CAD build for the part. Positions are in the model's coordinates, mm. A direction names the side the tool comes from. Coordinates: 2 decimals unless noted, no trailing zeros. Loops run counter-clockwise (first coordinate to the right, second up) from the corner with the lowest first, then second, coordinate; pieces in that order, holes last. Notation, with made-up numbers: (0, 20) -> (37, 20) arc R8 ccw to (37, 31) -> close; hole circle Ø5 at (20.5, -36.5). An arc over 180 degrees is marked (long way). Write each question's results on one line, items separated by ' | '.
from build123d import *

# Parameters (mm, degrees)
CROQUIS1_R              = 1.5
SALIENTE_EXTRUIR1_DEPTH = 10
CORTAR_EXTRUIR1_DEPTH   = 2
CHAFL_N2_SIZE           = 0.1
CHAFL_N3_SIZE           = 0.2
CHAFL_N3_SIZE2          = 0.346410162


with BuildPart() as part:
    # Croquis1 → Saliente-Extruir1 (new body)
    with BuildSketch(Plane(origin=(0, 0, 0), x_dir=(1, 0, 0), z_dir=(0, 1, 0))):
        Circle(CROQUIS1_R)
    extrude(amount=SALIENTE_EXTRUIR1_DEPTH)

    # Croquis2 → Cortar-Extruir1 (cut)
    with BuildSketch(Plane.XZ):
        Polygon((0.433012702, 0.75), (-0.433012702, 0.75), (-0.866025404, 0), (-0.433012702, -0.75), (0.433012702, -0.75), (0.866025404, 0), align=None)
    extrude(amount=-CORTAR_EXTRUIR1_DEPTH, mode=Mode.SUBTRACT)

    # Chaflán2
    chafl_n2_edges = [part.edges().sort_by_distance(p)[0] for p in [
        (-1.5, 0, 0),
    ]]
    chamfer(chafl_n2_edges, length=CHAFL_N2_SIZE)

    # Chaflán3
    chafl_n3_edges = [part.edges().sort_by_distance(p)[0] for p in [
        (-1.5, 10, 0),
    ]]
    chafl_n3_side = [part.faces().sort_by_distance(p)[0] for p in [
        (-1.5, 5.05, 0),
    ]]
    chamfer(chafl_n3_edges, length=CHAFL_N3_SIZE, length2=CHAFL_N3_SIZE2, reference=chafl_n3_side[0])


solid = part.part
1) Which spindle directions (+Z, -Z, +X, -X, +Y, -Y) get a long thin tool onto all of the face, cutting with end or side? Do faces 4 (the flat face through (0, 2, 0)), 5 (the flat face through (0, 10, 0)). Say none if no direction does.
Outcome:
face 4: -Y | face 5: +Z, -Z, +X, -X, +Y
2) Two-plate mould, pull along Z, no slides. Class faces 1 (the flat face through (0, 1, -0.75)), 2 (the cylindrical face through (-1.5, 4.88, -0.07)), 3 (the flat face through (0, 0, 1)): pulls with the +Z half, pulls with the -Z half, needs draft (parallel to the pull), parting line crosses it, or undercut.
Outcome:
face 1: undercut | face 2: parting line crosses it | face 3: needs draft
3) Slice it at A-A (y = 1). Write the cut outline in (x, z), then the cut area to 3 significant figures.
Outcome:
outline: circle Ø3 at (0, 0); hole (-0.87, 0) -> (-0.43, -0.75) -> (0.43, -0.75) -> (0.87, 0) -> (0.43, 0.75) -> (-0.43, 0.75) -> close | area: 5.12 mm^2
4) Slice it at B-B (x = 0). Write the cut outline in (y, z), then the cut area to 3 significant figures.
Outcome:
outline: (0, -1.4) -> (0.1, -1.5) -> (9.8, -1.5) -> (10, -1.15) -> (10, 1.15) -> (9.8, 1.5) -> (0.1, 1.5) -> (0, 1.4) -> (0, 0.75) -> (2, 0.75) -> (2, -0.75) -> (0, -0.75) -> close | area: 26.9 mm^2
5) Slice it at C-C (y = 5.5). Write the cut outline in (x, z), then the cut area to 3 significant figures.
Outcome:
outline: circle Ø3 at (0, 0) | area: 7.07 mm^2
6) Drill centre lines: L1, parallel to Z at x = -1.3, y = 6.5; L2, parallel to Y at x = 0.25, z = -0.55; L3, parallel to Z at x = -1, y = 1.5. Where is each one in solid material? Low to high. Write a range as from..to.
Outcome:
L1: z = -0.75..0.75 | L2: y = 2..10 | L3: z = -1.12..1.12
